```python
from build123d import *

# Parameters (mm, degrees)
SKETCH1_W                        = 64
SKETCH1_H                        = 64
BOSS_EXTRUDE1_DEPTH              = 6
F_4_6_4_6_DIAMETER_HOLE1_D       = 4.6
CBORE_FOR_M6_5_SHSS1_D           = 7.4
CBORE_FOR_M6_5_SHSS1_CBORE_D     = 10
CBORE_FOR_M6_5_SHSS1_CBORE_DEPTH = 2
M10X1_0_TAPPED_HOLE1_D           = 5.2
M10X1_0_TAPPED_HOLE1_CBORE_D     = 10
M10X1_0_TAPPED_HOLE1_CBORE_DEPTH = 2
BOSS_EXTRUDE4_START              = -32
SKETCH15_W                       = 28.2
SKETCH15_H                       = 29
BOSS_EXTRUDE4_DEPTH              = 6
BOSS_EXTRUDE5_START              = 32
SKETCH16_W                       = 28.2
SKETCH16_H                       = 29
BOSS_EXTRUDE5_DEPTH              = 6
CUT_EXTRUDE3_DEPTH               = 7
FILLET3_R                        = 10
FILLET4_R                        = 5


with BuildPart() as part:
    # Sketch1 → Boss-Extrude1 (new body)
    with BuildSketch(Plane(origin=(0, 6, 0), x_dir=(1, 0, 0), z_dir=(0, 1, 0))):
        Rectangle(SKETCH1_W, SKETCH1_H)
    extrude(amount=-BOSS_EXTRUDE1_DEPTH)

    # Ø4.6 (4.6) Diameter Hole1 (through all)
    with Locations(Plane(origin=(0, 0, 0), x_dir=(-1, 0, 0), z_dir=(0, -1, 0))):
        with Locations((0, 0)):
            Hole(F_4_6_4_6_DIAMETER_HOLE1_D / 2)

    # CBORE for M6.5 SHSS1 (through all)
    with Locations(Plane(origin=(0, 6, 0), x_dir=(1, 0, 0), z_dir=(0, 1, 0))):
        with Locations((21, 21), (-21, 21)):
            CounterBoreHole(CBORE_FOR_M6_5_SHSS1_D / 2, CBORE_FOR_M6_5_SHSS1_CBORE_D / 2, CBORE_FOR_M6_5_SHSS1_CBORE_DEPTH)

    # M10x1.0 Tapped Hole1 (through all)
    with Locations(Plane(origin=(0, 6, 0), x_dir=(1, 0, 0), z_dir=(0, 1, 0))):
        with Locations((-21, -21), (-21, 21), (21, -21)):
            CounterBoreHole(M10X1_0_TAPPED_HOLE1_D / 2, M10X1_0_TAPPED_HOLE1_CBORE_D / 2, M10X1_0_TAPPED_HOLE1_CBORE_DEPTH)

    # Sketch15 → Boss-Extrude4 (add)
    with BuildSketch(Plane(origin=(0, 0, 0), x_dir=(0, 0, -1), z_dir=(1, 0, 0)).offset(BOSS_EXTRUDE4_START)):
        with Locations((0, 14.5)):
            Rectangle(SKETCH15_W, SKETCH15_H)
        with BuildLine():
            Line((-11.3, 18.4), (-11.3, 24.9))
            ThreePointArc((-11.3, 24.9), (-10, 26.2), (-8.7, 24.9))
            Line((-8.7, 24.9), (-8.7, 18.4))
            ThreePointArc((-8.7, 18.4), (-10, 17.1), (-11.3, 18.4))
        make_face(mode=Mode.SUBTRACT)
        with BuildLine():
            Line((8.7, 8.25), (8.7, 14.75))
            ThreePointArc((8.7, 14.75), (10, 16.05), (11.3, 14.75))
            Line((11.3, 14.75), (11.3, 8.25))
            ThreePointArc((11.3, 8.25), (10, 6.95), (8.7, 8.25))
        make_face(mode=Mode.SUBTRACT)
    extrude(amount=BOSS_EXTRUDE4_DEPTH)

    # Sketch16 → Boss-Extrude5 (add)
    with BuildSketch(Plane(origin=(0, 0, 0), x_dir=(0, 0, -1), z_dir=(1, 0, 0)).offset(BOSS_EXTRUDE5_START)):
        with Locations((0, 14.5)):
            Rectangle(SKETCH16_W, SKETCH16_H)
        with BuildLine():
            Line((-11.3, 7.9), (-11.3, 14.4))
            ThreePointArc((-11.3, 14.4), (-10, 15.7), (-8.7, 14.4))
            Line((-8.7, 14.4), (-8.7, 7.9))
            ThreePointArc((-8.7, 7.9), (-10, 6.6), (-11.3, 7.9))
        make_face(mode=Mode.SUBTRACT)
        with BuildLine():
            Line((8.7, 18.4), (8.7, 24.9))
            ThreePointArc((8.7, 24.9), (10, 26.2), (11.3, 24.9))
            Line((11.3, 24.9), (11.3, 18.4))
            ThreePointArc((11.3, 18.4), (10, 17.1), (8.7, 18.4))
        make_face(mode=Mode.SUBTRACT)
    extrude(amount=-BOSS_EXTRUDE5_DEPTH)

    # Sketch17 → Cut-Extrude3 (cut, through all)
    with BuildSketch(Plane(origin=(0, 6, 0), x_dir=(1, 0, 0), z_dir=(0, 1, 0))):
        with BuildLine():
            Line((8, -5), (8, 5))
            ThreePointArc((8, 5), (10.5, 7.5), (13, 5))
            Line((13, 5), (13, -5))
            ThreePointArc((13, -5), (10.5, -7.5), (8, -5))
        make_face()
        with BuildLine():
            Line((18.5, -10), (18.5, 10))
            ThreePointArc((18.5, 10), (21, 12.5), (23.5, 10))
            Line((23.5, 10), (23.5, -10))
            ThreePointArc((23.5, -10), (21, -12.5), (18.5, -10))
        make_face()
        with BuildLine():
            Line((-5, -8), (5, -8))
            ThreePointArc((5, -8), (7.5, -10.5), (5, -13))
            Line((5, -13), (-5, -13))
            ThreePointArc((-5, -13), (-7.5, -10.5), (-5, -8))
        make_face()
        with BuildLine():
            Line((-10, -18.5), (10, -18.5))
            ThreePointArc((10, -18.5), (12.5, -21), (10, -23.5))
            Line((10, -23.5), (-10, -23.5))
            ThreePointArc((-10, -23.5), (-12.5, -21), (-10, -18.5))
        make_face()
        with BuildLine():
            Line((-8, 5), (-8, -5))
            ThreePointArc((-8, -5), (-10.5, -7.5), (-13, -5))
            Line((-13, -5), (-13, 5))
            ThreePointArc((-13, 5), (-10.5, 7.5), (-8, 5))
        make_face()
        with BuildLine():
            Line((-18.5, 10), (-18.5, -10))
            ThreePointArc((-18.5, -10), (-21, -12.5), (-23.5, -10))
            Line((-23.5, -10), (-23.5, 10))
            ThreePointArc((-23.5, 10), (-21, 12.5), (-18.5, 10))
        make_face()
        with BuildLine():
            Line((5, 8), (-5, 8))
            ThreePointArc((-5, 8), (-7.5, 10.5), (-5, 13))
            Line((-5, 13), (5, 13))
            ThreePointArc((5, 13), (7.5, 10.5), (5, 8))
        make_face()
        with BuildLine():
            Line((10, 18.5), (-10, 18.5))
            ThreePointArc((-10, 18.5), (-12.5, 21), (-10, 23.5))
            Line((-10, 23.5), (10, 23.5))
            ThreePointArc((10, 23.5), (12.5, 21), (10, 18.5))
        make_face()
    extrude(amount=-CUT_EXTRUDE3_DEPTH, mode=Mode.SUBTRACT)

    # Fillet3
    fillet3_edges = [part.edges().sort_by_distance(p)[0] for p in [
        (-32, 3, -32),
        (32, 3, -32),
        (32, 3, 32),
        (-32, 3, 32),
    ]]
    fillet(fillet3_edges, radius=FILLET3_R)

    # Fillet4
    fillet4_edges = [part.edges().sort_by_distance(p)[0] for p in [
        (-29, 29, -14.1),
        (-29, 29, 14.1),
        (29, 29, -14.1),
        (29, 29, 14.1),
    ]]
    fillet(fillet4_edges, radius=FILLET4_R)


solid = part.part
```
Work out the finished part from the listing and answer in its coordinate system (mm). A direction names the side the tool comes from. Coordinates: 2 decimals unless noted, no trailing zeros. Loops run counter-clockwise (first coordinate to the right, second up) from the corner with the lowest first, then second, coordinate; pieces in that order, holes last.
1) For faces 4 (the flat face through (-29, 12, -11.3)), 5 (the flat face through (-19, 4, 23)), 6 (the cylindrical face through (7.5, 3, 10.4)), 7 (the cylindrical face through (29, 17.1, -10)), determine the directions among +Z, -Z, +X, -X, +Y, -Y from which every point of the face is accessible in a straight line to the end or side of a thin tool.
Results:
face 4: -X
face 5: +Y
face 6: +Y, -Y
face 7: +X
2) Consider probe 1 along X at (y, z) = (1.9, 21); probe 2 along X at (y, z) = (4.7, -21). Determine where each line is inside the solid, lowest interval first.
Results:
probe 1: x = -32 to -23.6, -18.4 to -12.5, 12.5 to 18.4, 23.6 to 32
probe 2: x = -32 to -26, -16 to -12.5, 12.5 to 16, 26 to 32
3) Section C-C (x = 1) is taken. Give the vertices of the cut face in (y, z).
Results:
outline: (0, -32) - (6, -32) - (6, -23.5) - (0, -23.5) - close; (0, -18.5) - (6, -18.5) - (6, -13) - (0, -13) - close; (0, -8) - (6, -8) - (6, -2.07) - (0, -2.07) - close; (0, 2.07) - (6, 2.07) - (6, 8) - (0, 8) - close; (0, 13) - (6, 13) - (6, 18.5) - (0, 18.5) - close; (0, 23.5) - (6, 23.5) - (6, 32) - (0, 32) - close
4) Section B-B (y = 20.75) is taken. Give the vertices of the cut face in (x, z), plus the area to 3 significant figures.
Results:
outline: (-32, -14.1) - (-26, -14.1) - (-26, 8.7) - (-32, 8.7) - close; (-32, 11.3) - (-26, 11.3) - (-26, 14.1) - (-32, 14.1) - close; (26, -14.1) - (32, -14.1) - (32, -11.3) - (26, -11.3) - close; (26, -8.7) - (32, -8.7) - (32, 14.1) - (26, 14.1) - close
area: 307 mm2
5) For a pull along X with two mould halves and no side action, classify faces 1 (the flat face through (29, 22, -11.3)), 2 (the cylindrical face through (28.99, 2.96, 29.15)), 3 (the cylindrical face through (10.6, 3, 7.5)) as +X half, -X half, draft (parallel to the pull), parting line (faces both ways), or undercut.
Results:
face 1: draft
face 2: +X half
face 3: undercut
6) Section D-D (z = 20) is taken. Give the vertices of the cut face in (x, y), plus the area to 3 significant figures.
Results:
outline: (-32, 0) - (-23.4, 0) - (-23.4, 4) - (-25.9, 4) - (-25.9, 6) - (-32, 6) - close; (-18.6, 0) - (-12.29, 0) - (-12.29, 6) - (-16.1, 6) - (-16.1, 4) - (-18.6, 4) - close; (12.29, 0) - (18.6, 0) - (18.6, 4) - (16.1, 4) - (16.1, 6) - (12.29, 6) - close; (23.4, 0) - (32, 0) - (32, 6) - (25.9, 6) - (25.9, 4) - (23.4, 4) - close
area: 159 mm2
7) Flat-ended cylindrical pins translate along their axes: pin 1 (3 mm diameter, centred on x = -28, y = 12.5, fed in from +Z); pin 2 (6 mm diameter, centred on x = -21, z = 21, fed in from +Y); pin 3 (13 mm diameter, centred on x = -21, z = -21, fed in from +Y); pin 4 (5.5 mm diameter, centred on x = 0, z = 0, fed in from -Y). Find the tip coordinate at first contact, or state that the pin passes through.
Results:
pin 1: stops at z = 14.1
pin 2: stops at y = 4
pin 3: stops at y = 6
pin 4: stops at y = 0
8) Section A-A (z = 0) is taken. Give the vertices of the cut face in (x, y), plus the area to 3 significant figures.
Results:
outline: (-32, 0) - (-23.5, 0) - (-23.5, 6) - (-26, 6) - (-26, 29) - (-32, 29) - close; (-18.5, 0) - (-13, 0) - (-13, 6) - (-18.5, 6) - close; (-8, 0) - (-2.3, 0) - (-2.3, 6) - (-8, 6) - close; (2.3, 0) - (8, 0) - (8, 6) - (2.3, 6) - close; (13, 0) - (18.5, 0) - (18.5, 6) - (13, 6) - close; (23.5, 0) - (32, 0) - (32, 29) - (26, 29) - (26, 6) - (23.5, 6) - close
area: 512 mm2
